Build history of the part. All positions in model axes, mm. Face numbers are marked on the shaded views. A direction names the side the tool comes from. Give positions to 0.01 mm unless a question says otherwise; leave off trailing zeros. Order: outer loops, then holes, each group sorted by start corner. A loop starts at its lowest first (then second) coordinate and runs counter-clockwise, first axis right, second up. Notation, with made-up numbers: (65, 63) - (114, 63) arc R12 ccw to (114, 72) - close; hole circle Ø1 at (70.25, 21.25). An arc over 180 degrees is marked (long way). Use a Markdown table: item, result. Add a question column.
(1) Mould opens along X. For the marked faces 1, 2, 3 and 4 say: +X half, -X half, draft (parallel to the pull), parting line (faces both ways), or undercut.
(2) Slice it at A-A (y = 25.5). Count the separate pieces of the cut face and the enclosed holes in it, then the cut area to 3 significant figures.
(3) Which spindle directions (+Z, -Z, +X, -X, +Y, -Y) get a long thin tool onto all of the face, cutting with end or side? Do the marked faces 5 and 6. Say none if no direction does.
(4) Slice it at D-D (x = 0). Write the cut outline in (y, z), then the cut area to 3 significant figures.
(5) Flat gauge pins, fed straight in: pin 1 (1.8 mm diameter, centred on y = 25.5, z = 4, fed in from +X); pin 2 (5 mm diameter, centred on x = -18.5, z = 18.5, fed in from +Y). Where does each tip first touch, or does it go through?
(6) Wall check: line 1 (Y direction, x = 0, z = 3); line 2 (Y direction, x = 0, z = 9); line 3 (X direction, y = 2, z = 21.5). Give the ranges that are in metal, low to high.
(7) Slice it at C-C (y = 18.5). Write the cut outline in (x, z), then the cut area to 3 significant figures.
from build123d import *

# Parameters (mm, degrees)
SKETCH1_R               = 4.4
SKETCH1_R_2             = 12.196440552
BOSS_EXTRUDE1_DEPTH     = 24
SKETCH1_3_R             = 12.196440552
SKETCH1_3_R_2           = 1.5
SKETCH1_3_R_3           = 5
BOSS_EXTRUDE2_DEPTH     = 5
SKETCH2_R               = 1
CUT_EXTRUDE1_DEPTH      = 33.5
CUT_EXTRUDE1_DEPTH_BACK = 33.5


with BuildPart() as part:
    # Sketch1 → Boss-Extrude1 (new body)
    with BuildSketch(Plane.XY):
        Polygon((-32.5, 29.5), (-32.5, -17.5), (32.5, -17.5), (32.5, 29.5), (24, 29.5), (24, 17.5), (-24, 17.5), (-24, 29.5), align=None)
        with Locations((22.171280209, 0)):
            Circle(SKETCH1_R, mode=Mode.SUBTRACT)
        with Locations((-22.171280209, 0)):
            Circle(SKETCH1_R, mode=Mode.SUBTRACT)
        Circle(SKETCH1_R_2, mode=Mode.SUBTRACT)
    extrude(amount=BOSS_EXTRUDE1_DEPTH)

    # Sketch1<3> → Boss-Extrude2 (add)
    with BuildSketch(Plane.XY):
        Circle(SKETCH1_3_R)
        with Locations((-8, 0)):
            Circle(SKETCH1_3_R_2, mode=Mode.SUBTRACT)
        with Locations((0, -8)):
            Circle(SKETCH1_3_R_2, mode=Mode.SUBTRACT)
        with Locations((8, 0)):
            Circle(SKETCH1_3_R_2, mode=Mode.SUBTRACT)
        with Locations((0, 8)):
            Circle(SKETCH1_3_R_2, mode=Mode.SUBTRACT)
        Circle(SKETCH1_3_R_3, mode=Mode.SUBTRACT)
    extrude(amount=BOSS_EXTRUDE2_DEPTH)

    # Sketch2 → Cut-Extrude1 (cut, two sides)
    with BuildSketch(Plane(origin=(0, 0, 0), x_dir=(0, 0, -1), z_dir=(1, 0, 0))) as cut_extrude1_sk:
        with Locations((-20, 25.5)):
            Circle(SKETCH2_R)
        with Locations((-12, 25.5)):
            Circle(SKETCH2_R)
        with Locations((-4, 25.5)):
            Circle(SKETCH2_R)
    extrude(amount=CUT_EXTRUDE1_DEPTH, mode=Mode.SUBTRACT)
    extrude(cut_extrude1_sk.sketch, amount=-CUT_EXTRUDE1_DEPTH_BACK, mode=Mode.SUBTRACT)


solid = part.part
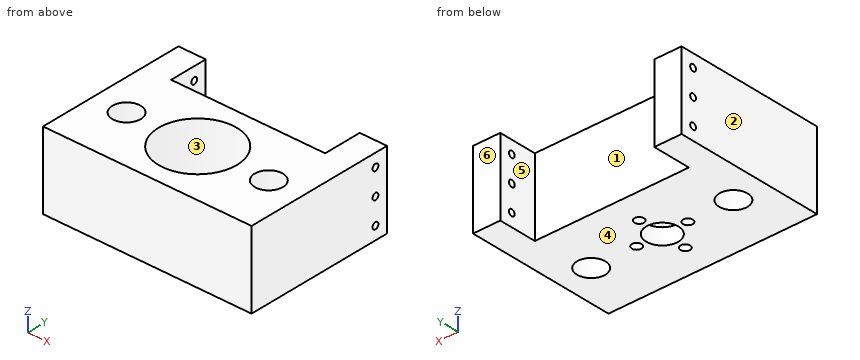
Solution:
| question | item | result |
|---|---|---|
| 1 | face 1 | undercut |
| 1 | face 2 | -X half |
| 1 | face 3 | undercut |
| 1 | face 4 | draft |
| 2 | separate pieces | 8 |
| 2 | enclosed holes | 0 |
| 2 | area | 306 mm2 |
| 3 | face 5 | +Z, -Z, +Y |
| 3 | face 6 | +Z, -Z, +X, -X, +Y |
| 4 | outline | (-17.5, 0) - (-9.5, 0) - (-9.5, 5) - (-12.2, 5) - (-12.2, 24) - (-17.5, 24) - close; (-6.5, 0) - (-5, 0) - (-5, 5) - (-6.5, 5) - close; (5, 0) - (6.5, 0) - (6.5, 5) - (5, 5) - close; (9.5, 0) - (17.5, 0) - (17.5, 24) - (12.2, 24) - (12.2, 5) - (9.5, 5) - close |
| 4 | area | 297 mm2 |
| 5 | pin 1 | through |
| 5 | pin 2 | y = 17.5 |
| 6 | line 1 | -17.5 to -9.5, -6.5 to -5, 5 to 6.5, 9.5 to 17.5 |
| 6 | line 2 | -17.5 to -12.2, 12.2 to 17.5 |
| 6 | line 3 | -32.5 to -26.09, -18.25 to -12.03, 12.03 to 18.25, 26.09 to 32.5 |
| 7 | outline | (-32.5, 0) - (-24, 0) - (-24, 24) - (-32.5, 24) - close; (24, 0) - (32.5, 0) - (32.5, 24) - (24, 24) - close |
| 7 | area | 408 mm2 |
